Geometry: final body of the model. Coordinates: model frame, mm. A direction names the side the tool comes from. Round coordinates to 2 decimals unless told otherwise and drop trailing zeros. Order: outer loops, then holes, each group sorted by start corner. A loop starts at its lowest first (then second) coordinate and runs counter-clockwise, first axis right, second up. Notation, with made-up numbers: M 83.5,80 L 101.5,80 A16 cw 101.5,108 Z; hole C 77.5,-28 d8. An arc over 180 degrees is marked long. Return JSON: item names as keys, results as strings. Group by question number.
Q1. Ray query, probe 1 along X at (y, z) = (29, -5.5); probe 2 along X at (y, z) = (5.5, -0.25); probe 3 along Y at (x, z) = (14.25, -8.25). Return the intervals inside material, ascending.
Q2. Contact query for flat-ended pins moving along their axis: pin 1 (3 mm diameter, centred on x = 12, z = -6.5, fed in from +Y); pin 2 (3 mm diameter, centred on x = 6, y = 8, fed in from +Z); pin 3 (4 mm diameter, centred on x = 6.5, z = -4.5, fed in from +Y). Output: stop coordinate, or through.
Q3. Cut plane C-C on z = -12.75. Output: boundary loops of the cut face in (x, y), and give its area (3 significant figures).
Q4. Mould query, pull axis X, two halves, no side actions, for faces 1 (the face through (16.99, 15.85, 1.52)), 2 (the face through (10, 5, -11)), 3 (the face through (9, 7, -1)), 4 (the face through (2.85, 16.01, 1.52)). Classes: released by +X, released by -X, zero draft, split by the parting line, or undercut.
Q5. Cut plane B-B on x = 1.5. Output: boundary loops of the cut face in (y, z), and give its area (3 significant figures).
Q6. Access query for faces 5 (the face through (14.5, 7.2, -1)), 6 (the face through (6, 7, 0)), 7 (the face through (13, 26, -2)). Directions: +Z, -Z, +X, -X, +Y, -Y. A direction counts if a zero-diameter tool reaches every point of the face in a straight line with its end or side. Return the directions, or none.
Autodesk Inventor part; units mm, degrees
ref_plane "YZ Plane" through (0, 0, 0) normal (1, 0, 0) x (0, 1, 0)
ref_plane "XZ Plane" through (0, 0, 0) normal (0, 1, 0) x (-1, 0, 0)
ref_plane "XY Plane" through (0, 0, 0) normal (0, 0, 1) x (1, 0, 0)
sketch "스케치1" plane through (0, 0, 0) normal (0, 0, 1) x (1, 0, 0)
  line L0 (0, 0) -> (20, 0)
  line L1 (20, 0) -> (20, 40)
  line L2 (20, 40) -> (0, 40)
  line L3 (0, 40) -> (0, 0)
  line L4 (0, 13) -> (20, 13)
  line L5 (10, 30) -> (10, 23) construction
  line L6 (7, 30) -> (7, 23)
  line L7 (13, 23) -> (13, 30)
  arc A0 (13, 30) -> (7, 30) centre (10, 30) ccw
  arc A1 (7, 23) -> (13, 23) centre (10, 23) ccw
  point P0 (10, 26.5)
  dimension "d0" = 20
  dimension "d1" = 40
  dimension "d2" = 27
  dimension "d4" = 7
  dimension "d5" = 13.5
  dimension "d6" = 10
  dimension "d7" = 3
extrude "돌출1" add sketch "스케치1" against normal blind 7
extrude "돌출2" add sketch "스케치1" along normal blind 3 contours L3 L2 L1 L4
fillet "모깎기1" radius 10 4 edges at (20, 40, -2) (0, 40, -2) (20, 13, 1.5) (0, 13, 1.5)
sketch "스케치2" plane through (0, 0, -7) normal (0, 0, -1) x (-1, 0, 0)
  line L0 (-20, 0) -> (-20, 23)
  line L1 (-20, 0) -> (0, 0)
  line L2 (-20, 0) -> (-20, 30)
  arc A0 (0, 30) -> (-20, 30) centre (-10, 30) ccw
  line L3 (0, 30) -> (0, 0)
  line L4 (0, 0) -> (-20, 0)
  line L5 (-13, 30) -> (-13, 23)
  arc A1 (-13, 23) -> (-7, 23) centre (-10, 23) ccw
  line L6 (-7, 23) -> (-7, 30)
  arc A2 (-7, 30) -> (-13, 30) centre (-10, 30) ccw
  line L7 (-20, 5) -> (0, 5)
  dimension "d14" = 5
extrude "돌출3" add sketch "스케치2" along normal blind 8 contours L0 L7 L3 L1
sketch "스케치3" plane through (0, 0, 0) normal (0, 0, 1) x (1, 0, 0)
  line L0 (2.6578, 12.3276) -> (17.6998, 12.3276) construction
  line L1 (17.6998, 12.3276) -> (17.6998, 1.5834) construction
  line L2 (17.6998, 1.5834) -> (2.6578, 1.5834) construction
  line L3 (2.6578, 1.5834) -> (2.6578, 12.3276) construction
  spline S0 degree 2 poles (9.6108, 7.1169) (9.6108, 4.4265) (8.0468, 1.9062) (6.4179, 1.9062) knots 0 0 0 1 2 2 2
  spline S1 degree 2 poles (6.4179, 1.9062) (4.7648, 1.9062) (3.217, 4.4751) (3.217, 7.1088) knots 0 0 0 1 2 2 2
  spline S2 degree 2 poles (3.217, 7.1088) (3.217, 9.8155) (4.781, 12.3195) (6.4179, 12.3195) knots 0 0 0 1 2 2 2
  spline S3 degree 2 poles (6.4179, 12.3195) (8.063, 12.3195) (9.6108, 9.7263) (9.6108, 7.1169) knots 0 0 0 1 2 2 2
  spline S4 degree 2 poles (7.8928, 4.0699) (8.0873, 4.5643) (8.2494, 6.0878) (8.2494, 7.1169) knots 0 0 0 1 2 2 2
  spline S5 degree 2 poles (8.2494, 7.1169) (8.2494, 8.1461) (8.0873, 9.6615) (7.8847, 10.1721) knots 0 0 0 1 2 2 2
  spline S6 degree 2 poles (7.8847, 10.1721) (7.6821, 10.6826) (6.9771, 11.2093) (6.4179, 11.2093) knots 0 0 0 1 2 2 2
  spline S7 degree 2 poles (6.4179, 11.2093) (5.8588, 11.2093) (5.1375, 10.6826) (4.9268, 10.1558) knots 0 0 0 1 2 2 2
  spline S8 degree 2 poles (4.9268, 10.1558) (4.7242, 9.6453) (4.5784, 8.0894) (4.5784, 7.1088) knots 0 0 0 1 2 2 2
  spline S9 degree 2 poles (4.5784, 7.1088) (4.5784, 6.0554) (4.708, 4.6453) (4.9187, 4.0943) knots 0 0 0 1 2 2 2
  spline S10 degree 2 poles (4.9187, 4.0943) (5.1132, 3.5756) (5.8345, 3.0165) (6.4179, 3.0165) knots 0 0 0 1 2 2 2
  spline S11 degree 2 poles (6.4179, 3.0165) (6.969, 3.0165) (7.6902, 3.5432) (7.8928, 4.0699) knots 0 0 0 1 2 2 2
  spline S12 degree 2 poles (13.5897, 11.1688) (13.2251, 11.1688) (12.5038, 10.9905) (12.1554, 10.8528) knots 0 0 0 1 2 2 2
  spline S13 degree 2 poles (12.1554, 10.8528) (11.8312, 10.715) (11.3531, 10.4233) (11.1667, 10.2936) knots 0 0 0 1 2 2 2
  line L4 (11.1667, 10.2936) -> (11.0857, 10.2936)
  line L5 (11.0857, 10.2936) -> (11.0857, 11.7118)
  spline S14 degree 2 poles (11.0857, 11.7118) (11.5233, 11.9468) (13.0225, 12.3276) (13.6951, 12.3276) knots 0 0 0 1 2 2 2
  spline S15 degree 2 poles (13.6951, 12.3276) (14.3758, 12.3276) (15.3888, 12.0521) (15.802, 11.7604) knots 0 0 0 1 2 2 2
  spline S16 degree 2 poles (15.802, 11.7604) (16.2396, 11.4443) (16.6935, 10.5286) (16.6935, 9.9127) knots 0 0 0 1 2 2 2
  spline S17 degree 2 poles (16.6935, 9.9127) (16.6935, 9.0862) (15.6076, 7.8382) (14.8458, 7.6761) knots 0 0 0 1 2 2 2
  line L6 (14.8458, 7.6761) -> (14.8458, 7.5789)
  spline S18 degree 2 poles (14.8458, 7.5789) (15.1618, 7.514) (15.8831, 7.2223) (16.191, 6.9306) knots 0 0 0 1 2 2 2
  spline S19 degree 2 poles (16.191, 6.9306) (16.499, 6.6469) (16.8879, 5.7393) (16.8879, 5.0829) knots 0 0 0 1 2 2 2
  spline S20 degree 2 poles (16.8879, 5.0829) (16.8879, 4.4103) (16.426, 3.2677) (16.0046, 2.8301) knots 0 0 0 1 2 2 2
  spline S21 degree 2 poles (16.0046, 2.8301) (15.567, 2.3763) (14.3272, 1.9062) (13.5411, 1.9062) knots 0 0 0 1 2 2 2
  spline S22 degree 2 poles (13.5411, 1.9062) (12.7875, 1.9062) (11.3126, 2.2709) (10.8101, 2.5221) knots 0 0 0 1 2 2 2
  line L7 (10.8101, 2.5221) -> (10.8101, 3.9403)
  line L8 (10.8101, 3.9403) -> (10.9074, 3.9403)
  spline S23 degree 2 poles (10.9074, 3.9403) (11.3288, 3.6323) (12.755, 3.0651) (13.4601, 3.0651) knots 0 0 0 1 2 2 2
  spline S24 degree 2 poles (13.4601, 3.0651) (13.8734, 3.0651) (14.6999, 3.3244) (14.9755, 3.6242) knots 0 0 0 1 2 2 2
  spline S25 degree 2 poles (14.9755, 3.6242) (15.2429, 3.9241) (15.5265, 4.6372) (15.5265, 5.1802) knots 0 0 0 1 2 2 2
  spline S26 degree 2 poles (15.5265, 5.1802) (15.5265, 5.7231) (15.2105, 6.4281) (14.9268, 6.6307) knots 0 0 0 1 2 2 2
  spline S27 degree 2 poles (14.9268, 6.6307) (14.6432, 6.8333) (13.8734, 6.9873) (13.4195, 6.9873) knots 0 0 0 1 2 2 2
  line L9 (13.4195, 6.9873) -> (12.8523, 6.9873)
  line L10 (12.8523, 6.9873) -> (12.8523, 8.0975)
  line L11 (12.8523, 8.0975) -> (13.298, 8.0975)
  spline S28 degree 2 poles (13.298, 8.0975) (14.1975, 8.0975) (15.332, 8.9565) (15.332, 9.775) knots 0 0 0 1 2 2 2
  spline S29 degree 2 poles (15.332, 9.775) (15.332, 10.1558) (15.0403, 10.6988) (14.8053, 10.8609) knots 0 0 0 1 2 2 2
  spline S30 degree 2 poles (14.8053, 10.8609) (14.5541, 11.031) (13.9382, 11.1688) (13.5897, 11.1688) knots 0 0 0 1 2 2 2
  point P0 (0, 0)
extrude "돌출4" cut sketch "스케치3" against normal blind 1
properties part number "1번부품"
Result sheet:
{
 "1": {"probe 1": "x = 0 to 7, 13 to 20", "probe 2": "x = 0 to 3.3, 4.63 to 8.19, 9.53 to 15.51, 16.87 to 20", "probe 3": "y = 0 to 5"},
 "2": {"pin 1": "stops at y = 39.99", "pin 2": "stops at z = 0", "pin 3": "stops at y = 39.89"},
 "3": {"outline": "M 0,0 L 20,0 L 20,5 L 0,5 Z", "area": "100 mm²"},
 "4": {"face 1": "released by +X", "face 2": "zero draft", "face 3": "undercut", "face 4": "released by -X"},
 "5": {"outline": "M 0,-15 L 5,-15 L 5,-7 L 35.27,-7 L 35.27,3 L 17.73,3 L 17.73,0 L 0,0 Z", "area": "339 mm²"},
 "6": {"face 5": "+Z", "face 6": "+Z, +X, -X, -Y", "face 7": "+Z, -Z"}
}
